Work out the finished part from the listing and answer in its coordinate system (mm). A direction names the side the tool comes from. Give positions to 0.01 mm unless a question says otherwise; leave off trailing zeros. Order: outer loops, then holes, each group sorted by start corner. A loop starts at its lowest first (then second) coordinate and runs counter-clockwise, first axis right, second up. Notation, with made-up numbers: (-36.5, -32) - (18.5, -32) arc R18 ccw to (18.5, -2) - close; hole circle Ø9 at (-35, 33.5). An arc over 180 degrees is marked (long way). Return JSON: item names as keys, results as strings. Group by question number.
from build123d import *

# Parameters (mm, degrees)
F0_W     = 66.8018609285
F0_H     = 44.45
F1_DEPTH = 25.4
F3_DEPTH = 12.7
F5_DEPTH = 19.05


with BuildPart() as f1:
    # F0 (on Front) → F1 (new body)
    with BuildSketch(Plane.XZ):
        with Locations((-6.9442056119, 13.2829286516)):
            Rectangle(F0_W, F0_H)
    extrude(amount=F1_DEPTH)

    # F2 (on face) → F3 (cut)
    with BuildSketch(Plane.XZ.offset(25.4)):
        Polygon((26.4567248523, 35.5079286516), (-21.2951360762, 35.5079286516), (4.1048639238, -8.9420713484), (26.4567248523, -8.9420713484), align=None)
    extrude(amount=-F3_DEPTH, mode=Mode.SUBTRACT)

    # F4 (on face) → F5 (cut)
    with BuildSketch(Plane.XZ.offset(25.4)):
        with BuildLine():
            Line((-3.6320969141, 4.5976101178), (-15.4953949278, 25.3583816418))
            ThreePointArc((-15.4953949278, 25.3583816418), (-23.3260269454, 7.1138352944), (-3.6320969141, 4.5976101178))
        make_face()
    extrude(amount=-F5_DEPTH, mode=Mode.SUBTRACT)


solid = f1.part
1. A tool of negligible diameter and unlimited length cuts with its end or side. For faces 5 (the flat face through (-18.436, -19.139, 30.504)), 6 (the cylindrical face through (-23.482, -16.008, 7.395)), 7 (the flat face through (-15, -13, -8.942)), from which of +Z, -Z, +X, -X, +Y, -Y can it reach the whole face along a straight path? Write none if from no direction.
2. Each of these flat-tipped pins is pushed along its axis until it touches: pin 1 (5 mm diameter, centred on x = 16.5, y = -17, fed in from -Z); pin 2 (6 mm diameter, centred on x = 19.5, z = 29, fed in from -Y). Where does it stop, or does it pass through?
3. Consider probe 1 along X at (y, z) = (-7, 15); probe 2 along Y at (x, z) = (-12.5, 30.5); probe 3 along Z at (x, y) = (-18.5, -20.5). Determine where each line is inside the solid, lowest interval first. Write a range as from..to.
4. The part is cut by section B-B (x = -14). Give the vertices of the cut face in (y, z), and give its area (4 significant figures).
5. Determine the mould class of faces 1 (the flat face through (-9.48, -9.57, 14.83)), 2 (the flat face through (8, -12.7, 19)), 3 (the flat face through (0.182, -19.139, -2.077)), 4 (the flat face through (-14, -6.35, 11)) for opening direction Z: released by +Z, released by -Z, zero draft, split by the parting line, or undercut.
6. The part is cut by section D-D (y = -14.5). Give the vertices of the cut face in (x, z).
7. The part is cut by section C-C (z = 7). Give the vertices of the cut face in (x, y).
8. The part is cut by section A-A (y = -11.25). Give the vertices of the cut face in (x, z).
Answers:
{
 "1": {"face 5": "+Z, +X, -Y", "face 6": "-Y", "face 7": "-Z, +X, -X, +Y, -Y"},
 "2": {"pin 1": "passes through", "pin 2": "stops at y = -12.7"},
 "3": {"probe 1": "x = -40.35..-24.85, -9.58..26.46", "probe 2": "y = -12.7..0", "probe 3": "z = -8.94..2.38, 24.19..30.62"},
 "4": {"outline": "(-25.4, -8.94) - (0, -8.94) - (0, 35.51) - (-12.7, 35.51) - (-12.7, 22.74) - (-6.35, 22.74) - (-6.35, 0.94) - (-25.4, 0.94) - close", "area": "551.5 mm^2"},
 "5": {"face 1": "undercut", "face 2": "zero draft", "face 3": "released by +Z", "face 4": "undercut"},
 "6": {"outline": "(-40.35, -8.94) - (4.1, -8.94) - (-3.63, 4.6) arc R12.43 cw (long way) to (-15.5, 25.36) - (-21.3, 35.51) - (-40.35, 35.51) - close"},
 "7": {"outline": "(-40.35, -25.4) - (-23.26, -25.4) - (-23.26, -6.35) - (-5, -6.35) - (-5, -12.7) - (26.46, -12.7) - (26.46, 0) - (-40.35, 0) - close"},
 "8": {"outline": "(-40.35, -8.94) - (26.46, -8.94) - (26.46, 35.51) - (-40.35, 35.51) - close; hole (-15.5, 25.36) arc R12.43 ccw (long way) to (-3.63, 4.6) - close"}
}
